Work out the finished part from the listing and answer in its coordinate system (mm). A direction names the side the tool comes from. Coordinates: 2 decimals unless noted, no trailing zeros. Order: outer loops, then holes, each group sorted by start corner. A loop starts at its lowest first (then second) coordinate and runs counter-clockwise, first axis right, second up. Notation, with made-up numbers: M 43,69 L 84,69 A13 ccw 84,84 Z; hole C -38.75,59 d5. An arc over 180 degrees is marked long. Use a Markdown table: item, result.
from build123d import *

# Parameters (mm, degrees)
F0_W     = 910
F0_H     = 500
F0_W_2   = 880
F0_H_2   = 470
F1_DEPTH = 50
F2_DEPTH = 15
F3_W     = 880
F3_H     = 45
F3_H_2   = 20
F4_DEPTH = 15


with BuildPart() as f1:
    # F0 (on Top) → F1 (new body)
    with BuildSketch(Plane.XY):
        Rectangle(F0_W, F0_H)
        Rectangle(F0_W_2, F0_H_2, mode=Mode.SUBTRACT)
    extrude(amount=F1_DEPTH)

    # F0 (on Top) → F2 (join)
    with BuildSketch(Plane.XY):
        Rectangle(F0_W_2, F0_H_2)
    extrude(amount=F2_DEPTH)

    # F3 (on face) → F4 (cut, through all)
    with BuildSketch(Plane.XY.offset(15)):
        with Locations((0, 142.5)):
            Rectangle(F3_W, F3_H)
        with Locations((0, 47.5)):
            Rectangle(F3_W, F3_H)
        with Locations((0, -47.5)):
            Rectangle(F3_W, F3_H)
        with Locations((0, -142.5)):
            Rectangle(F3_W, F3_H)
        with Locations((0, 225)):
            Rectangle(F3_W, F3_H_2)
        with Locations((0, -225)):
            Rectangle(F3_W, F3_H_2)
    extrude(amount=-F4_DEPTH, mode=Mode.SUBTRACT)


solid = f1.part
(1) Determine the mould class of faces 1 (the flat face through (-137, -240, 50)), 2 (the flat face through (440, -3, 31)), 3 (the flat face through (-6, -95, 15)), 4 (the flat face through (-6, 250, 25)) for opening direction Y: pulls with the +Y half, pulls with the -Y half, needs draft (parallel to the pull), parting line crosses it, or undercut.
Conclusion:
| item | result |
|---|---|
| face 1 | needs draft |
| face 2 | undercut |
| face 3 | undercut |
| face 4 | pulls with the +Y half |
(2) Given P1, Ø15, axis at x = -216.5, y = 177.5, coming from the +Z side; P2, Ø1.5, axis at x = -183.5, y = 164, coming from the -Z side, each flat-ended and moving along its own axis, determine where each tip first touches the part or whether it passes through.
Conclusion:
| item | result |
|---|---|
| P1 | z = 15 |
| P2 | through |
(3) A cutting plane is placed at B-B (z = 29). Determine the outline of the cut face in (x, y), then the cut area to 3 significant figures.
Conclusion:
| item | result |
|---|---|
| outline | M -455,-250 L 455,-250 L 455,250 L -455,250 Z; hole M -440,-235 L 440,-235 L 440,235 L -440,235 Z |
| area | 41,400 mm2 |
(4) Which of the six approach directions +Z, -Z, +X, -X, +Y, -Y give full straight-line access (tool end or side, diameter ignored) to faces 5 (the flat face through (-6, 235, 25)), 6 (the flat face through (-440, -3, 31)), 7 (the flat face through (-6, -250, 25))?
Conclusion:
| item | result |
|---|---|
| face 5 | +Z, -Z |
| face 6 | +Z |
| face 7 | +Z, -Z, +X, -X, -Y |
(5) A cutting plane is placed at A-A (y = -55). Determine the outline of the cut face in (x, z), then the cut area to 3 significant figures.
Conclusion:
| item | result |
|---|---|
| outline | M -455,0 L -440,0 L -440,50 L -455,50 Z; M 440,0 L 455,0 L 455,50 L 440,50 Z |
| area | 1,500 mm2 |
(6) Straight lines are drawn through the part: L1, parallel to X at y = -18, z = 48; L2, parallel to Y at x = -128.5, z = 30.5; L3, parallel to Z at x = 361, y = -196.5. For each, find the intervals that lie inside material, in ascending order.
Conclusion:
| item | result |
|---|---|
| L1 | -455 to -440, 440 to 455 |
| L2 | -250 to -235, 235 to 250 |
| L3 | 0 to 15 |
(7) A cutting plane is placed at D-D (y = -2). Determine the outline of the cut face in (x, z).
Conclusion:
| item | result |
|---|---|
| outline | M -455,0 L 455,0 L 455,50 L 440,50 L 440,15 L -440,15 L -440,50 L -455,50 Z |
(8) A cutting plane is placed at C-C (x = -382). Determine the outline of the cut face in (y, z), then the cut area to 3 significant figures.
Conclusion:
| item | result |
|---|---|
| outline | M -250,0 L -235,0 L -235,50 L -250,50 Z; M -215,0 L -165,0 L -165,15 L -215,15 Z; M -120,0 L -70,0 L -70,15 L -120,15 Z; M -25,0 L 25,0 L 25,15 L -25,15 Z; M 70,0 L 120,0 L 120,15 L 70,15 Z; M 165,0 L 215,0 L 215,15 L 165,15 Z; M 235,0 L 250,0 L 250,50 L 235,50 Z |
| area | 5,250 mm2 |
